Autodesk Inventor part; units mm, degrees
ref_plane "YZ Plane" through (0, 0, 0) normal (1, 0, 0) x (0, 1, 0)
ref_plane "XZ Plane" through (0, 0, 0) normal (0, 1, 0) x (-1, 0, 0)
ref_plane "XY Plane" through (0, 0, 0) normal (0, 0, 1) x (1, 0, 0)
ref_plane "Arbeitsebene1" through (0, 0, 0) normal (0, 0, 1) x (1, 0, 0)
sketch "Skizze1" plane through (0, 0, 0) normal (0, 0, 1) x (1, 0, 0)
  line L0 (-12.5, 37) -> (-12.5, -37)
  line L1 (-12.5, -37) -> (12.5, -37)
  line L2 (12.5, -37) -> (12.5, 37)
  line L3 (12.5, 37) -> (-12.5, 37)
  circle A0 centre (8.5, 30) radius 1.4
  circle A1 centre (-8.5, 30) radius 1.4
  circle A2 centre (-8.5, -30) radius 1.4
  circle A3 centre (8.5, -30) radius 1.4
  line L4 (9.25, 9.25) -> (9.25, -9.25)
  line L5 (9.25, -9.25) -> (-9.25, -9.25)
  line L6 (-9.25, -9.25) -> (-9.25, 9.25)
  line L7 (-9.25, 9.25) -> (9.25, 9.25)
  arc A4 (0.75, 23.146) -> (-0.75, 23.146) centre (0, 25) ccw
  line L8 (0.75, -23.146) -> (0.75, 23.146)
  arc A5 (-0.75, -23.146) -> (0.75, -23.146) centre (0, -25) ccw
  line L9 (-0.75, 23.146) -> (-0.75, -23.146)
  point P0 (0, 0)
extrude "Extrusion1" add sketch "Skizze1" along normal blind 0.4 contours L3 L2 L1 L0 | L4 L5 L8 L7 | L9 L5 L6 L7
sketch "Skizze2" plane through (0, 0, 0.4) normal (0, 0, 1) x (1, 0, 0)
  arc A0 (0.75, 23.146) -> (-0.75, 23.146) centre (0, 25) ccw
  line L0 (-12.5, -37) -> (12.5, -37)
  line L1 (12.5, -37) -> (12.5, 37)
  line L2 (12.5, 37) -> (-12.5, 37)
  line L3 (-12.5, 37) -> (-12.5, -37)
  circle A1 centre (8.5, -30) radius 1.4
  circle A2 centre (-8.5, -30) radius 1.4
  circle A3 centre (-8.5, 30) radius 1.4
  circle A4 centre (8.5, 30) radius 1.4
  line L4 (0.75, 23.146) -> (0.75, -23.146)
  arc A5 (-0.75, -23.146) -> (0.75, -23.146) centre (0, -25) ccw
  line L5 (-0.75, -23.146) -> (-0.75, 23.146)
  arc A6 (0.75, 23.146) -> (-0.75, 23.146) centre (0, 25) ccw
  circle A7 centre (0, 25) radius 2.5
  line L6 (-9.25, 9.25) -> (9.25, 9.25)
  line L7 (9.25, -9.25) -> (-9.25, -9.25)
  line L8 (0.75, 23.146) -> (0.75, -23.146)
  line L9 (0.75, 22.6152) -> (-0.75, 22.6152)
  line L10 (-0.75, 22.6152) -> (-0.75, 9.25)
  line L11 (-0.75, 9.25) -> (0.75, 9.25)
  line L12 (0.75, 9.25) -> (0.75, 22.6152)
  line L13 (-0.75, -23.146) -> (-0.75, 23.146)
  line L14 (0.75, -9.25) -> (-0.75, -9.25)
  line L15 (-0.75, -9.25) -> (-0.75, -23.146)
  line L16 (-0.75, -23.146) -> (0.75, -23.146)
  line L17 (0.75, -23.146) -> (0.75, -9.25)
  arc A8 (-0.75, -23.146) -> (0.75, -23.146) centre (0, -25) ccw
  circle A9 centre (0, -25) radius 2.5
  line L18 (0.75, 9.25) -> (-0.75, 9.25)
  line L19 (-0.75, 9.25) -> (-0.75, 7.25)
  line L20 (-0.75, 7.25) -> (0.75, 7.25)
  line L21 (0.75, 7.25) -> (0.75, 9.25)
  line L22 (0.75, -9.25) -> (-0.75, -9.25)
  line L23 (-0.75, -9.25) -> (-0.75, -7.25)
  line L24 (-0.75, -7.25) -> (0.75, -7.25)
  line L25 (0.75, -7.25) -> (0.75, -9.25)
  point P0 (0, 0)
  point P1 (0.75, -9.25)
  point P2 (0.75, 9.25)
  point P3 (0.75, -7.25)
  dimension "d2" = 5
  dimension "d11" = 1.5
  dimension "d12" = 2
  dimension "d13" = 2
extrude "Extrusion2" add sketch "Skizze2" along normal blind 0.4 contours L4 L9 L5 A0 | A0 L5 A7 L4 | L4 L6 L5 A7 | A7 L9 | L4 L20 L5 L6 | L4 L7 L5 L24 | L4 A9 L5 L7 | A9 L5 A5 L4 | L4 L16 L5 A9 | A5 L16 | L3 L2 L1 L0
sketch "Skizze3" plane through (0, 0, 0.8) normal (0, 0, 1) x (1, 0, 0)
  arc A0 (0.75, 23.146) -> (-0.75, 23.146) centre (0, 25) ccw
  arc A1 (-0.75, -23.146) -> (0.75, -23.146) centre (0, -25) ccw
  arc A2 (0.75, 23.146) -> (-0.75, 23.146) centre (0, 25) ccw
  circle A3 centre (0, 25) radius 2.5
  circle A4 centre (0, -25) radius 2.5
  point P0 (0, 0)
  dimension "d5" = 5
  dimension "d6" = 5
extrude "Extrusion3" add sketch "Skizze3" along normal blind 5
sketch "Skizze4" plane through (0, 0, 0.8) normal (0, 0, 1) x (1, 0, 0)
  circle A0 centre (0, -25) radius 2.5
  circle A1 centre (0, 25) radius 2.5
  line L0 (12.5, -37) -> (12.5, 37)
  line L1 (12.5, 37) -> (-12.5, 37)
  line L2 (-12.5, 37) -> (-12.5, -37)
  line L3 (-12.5, -37) -> (12.5, -37)
  line L4 (-0.75, -7.25) -> (-0.75, 7.25)
  line L5 (0.75, 7.25) -> (0.75, -7.25)
  circle A2 centre (8.5, -30) radius 1.4
  circle A3 centre (-8.5, -30) radius 1.4
  circle A4 centre (-8.5, 30) radius 1.4
  circle A5 centre (8.5, 30) radius 1.4
  line L6 (-9.25, -9.25) -> (9.25, -9.25)
  line L7 (9.25, -9.25) -> (9.25, 9.25)
  line L8 (9.25, 9.25) -> (-9.25, 9.25)
  line L9 (-9.25, 9.25) -> (-9.25, -9.25)
  line L10 (-9.25, -9.25) -> (9.25, 9.25) construction
  line L11 (9.25, -9.25) -> (-9.25, 9.25) construction
  line L12 (0.75, -7.25) -> (-0.75, -7.25)
  line L13 (-0.75, 7.25) -> (0.75, 7.25)
  point P0 (0, 0)
  dimension "d9" = 18.5
  dimension "d10" = 18.5
extrude "Extrusion4" cut sketch "Skizze4" against normal blind 0.3 contours L9 L8 L7 L6
equation "\"d7\" = d6"
properties part number "40_microfluidic_chip_lightsheet_layer1_negative_v0"
The model under review builds one solid part; all positions refer to its coordinate system, in mm. A direction names the side the tool comes from. Round coordinates to 2 decimals unless told otherwise and drop trailing zeros. Order: outer loops, then holes, each group sorted by start corner. A loop starts at its lowest first (then second) coordinate and runs counter-clockwise, first axis right, second up. Notation, with made-up numbers: (89, 61) -> (128, 61) arc R28 cw to (128, 94) -> close; hole circle Ø11 at (13.25, 36). An arc over 180 degrees is marked (long way). Return JSON: item names as keys, results as strings.
1. The part is to be moulded in two halves that separate along Y. For faces 1 (the face through (-8.68, 28.61, 0.39)), 2 (the face through (0, -25, 5.8)), say which applies: +Y half, -Y half, draft (parallel to the pull), parting line (faces both ways), or undercut.
Answer block:
{"face 1": "undercut", "face 2": "draft"}
2. Insertion check: P1, Ø2.5, axis at x = -8.5, y = 30, coming from the -Z side; P2, Ø3, axis at x = 10, y = 25.5, coming from the +Z side; P3, Ø2, axis at x = -3, z = 2.5, coming from the +Y side. Each pin has a flat end and moves straight along its axis. Give the tip position at first contact, or say it passes through.
Answer block:
{"P1": "passes through", "P2": "stops at z = 0.8", "P3": "stops at y = 26.5"}
3. Take a section at C-C (x = 8.5). Write out the cut boundary in (y, z).
Answer block:
{"outline": "(-37, 0) -> (-31.4, 0) -> (-31.4, 0.8) -> (-37, 0.8) -> close; (-28.6, 0) -> (28.6, 0) -> (28.6, 0.8) -> (9.25, 0.8) -> (9.25, 0.5) -> (-9.25, 0.5) -> (-9.25, 0.8) -> (-28.6, 0.8) -> close; (31.4, 0) -> (37, 0) -> (37, 0.8) -> (31.4, 0.8) -> close"}
4. Take a section at B-B (x = 0). Write out the cut boundary in (y, z), then the cut area to 3 significant figures.
Answer block:
{"outline": "(-37, 0) -> (-27, 0) -> (-27, 0.4) -> (-7.25, 0.4) -> (-7.25, 0.5) -> (-9.25, 0.5) -> (-9.25, 0.8) -> (-22.5, 0.8) -> (-22.5, 5.8) -> (-27.5, 5.8) -> (-27.5, 0.8) -> (-37, 0.8) -> close; (7.25, 0.4) -> (27, 0.4) -> (27, 0) -> (37, 0) -> (37, 0.8) -> (27.5, 0.8) -> (27.5, 5.8) -> (22.5, 5.8) -> (22.5, 0.8) -> (9.25, 0.8) -> (9.25, 0.5) -> (7.25, 0.5) -> close", "area": "80.6 mm²"}
5. For L1, parallel to Y at x = -8.5, z = 0.2; L2, parallel to X at y = -25, z = 0.2; L3, parallel to Z at x = 10.25, y = -3, list the stretches that pass through material, from the lowest coordinate up. Write a range as [from, to].
Answer block:
{"L1": "y = [-37, -31.4], [-28.6, 28.6], [31.4, 37]", "L2": "x = [-12.5, -2], [2, 12.5]", "L3": "z = [0, 0.8]"}
6. Take a section at A-A (y = 30). Write out the cut boundary in (x, z), then the cut area to 3 significant figures.
Answer block:
{"outline": "(-12.5, 0) -> (-9.9, 0) -> (-9.9, 0.8) -> (-12.5, 0.8) -> close; (-7.1, 0) -> (7.1, 0) -> (7.1, 0.8) -> (-7.1, 0.8) -> close; (9.9, 0) -> (12.5, 0) -> (12.5, 0.8) -> (9.9, 0.8) -> close", "area": "15.5 mm²"}
7. Take a section at D-D (z = 1.6). Write out the cut boundary in (x, y), then the cut area to 3 significant figures.
Answer block:
{"outline": "circle Ø5 at (0, -25); circle Ø5 at (0, 25)", "area": "39.3 mm²"}
8. For faces 3 (the face through (-2, 0, 0.5)), 4 (the face through (0, 19, 0.4)), 5 (the face through (3, 1, 0)), list the 3-axis set-ups (+Z, -Z, +X, -X, +Y, -Y) from which the entire face can be reached by the end or side of a thin tool; tool diameter is ignored.
Answer block:
{"face 3": "+Z", "face 4": "-Z", "face 5": "-Z, +X, -X, +Y, -Y"}
